The drawing under review shows one solid part. Ordinate dimensions are in mm from its lowest x, y, z. Coordinates: 2 decimals unless noted, no trailing zeros. Order: outer loops, then holes, each group sorted by start corner. A loop starts at its lowest first (then second) coordinate and runs counter-clockwise, first axis right, second up. Notation, with made-up numbers: (-15, 45.5) - (39, 45.5) arc R19 cw to (39, 50.5) - close; hole circle Ø9 at (61.5, 78.5). An arc over 180 degrees is marked (long way). Answer in a Markdown table with one row per item.
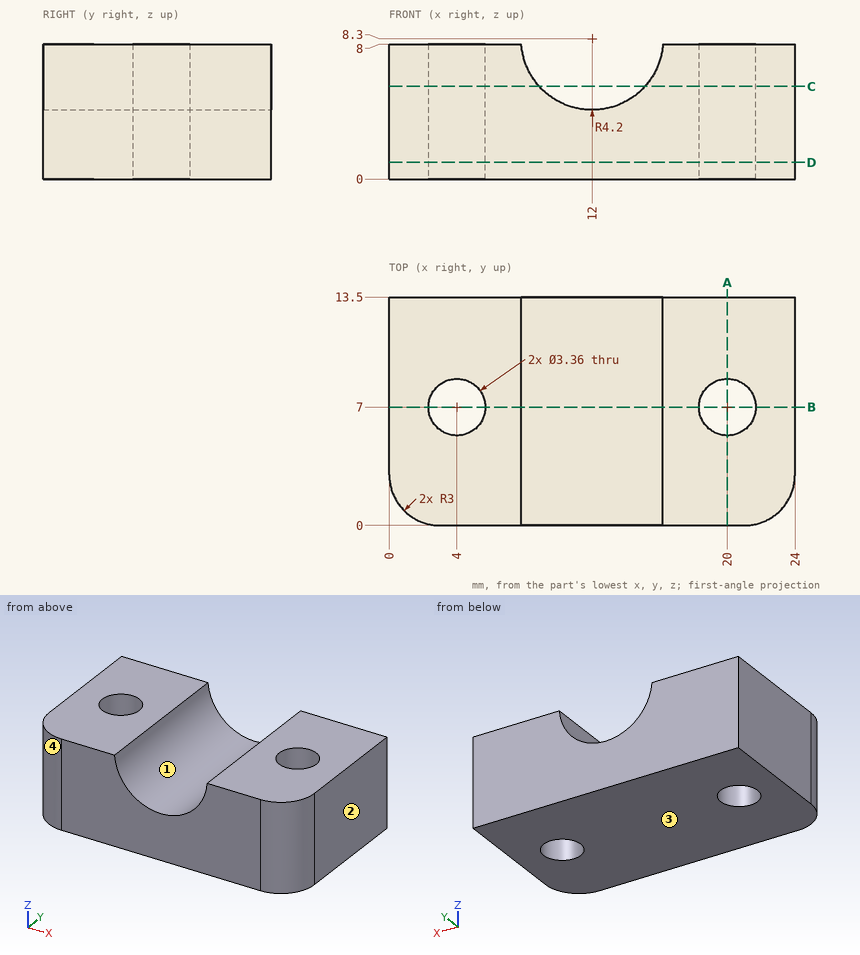
Item 1: Mouldability with a two-part tool opening along X and no side actions: class the marked faces 1, 2, 3 and 4 as +X half, -X half, draft (parallel to the pull), parting line (faces both ways), or undercut.
Check values:
| item | result |
|---|---|
| face 1 | undercut |
| face 2 | +X half |
| face 3 | draft |
| face 4 | -X half |
Item 2: To check wall thickness, follow line 1 (X direction, y = 7, z = 4); line 2 (X direction, y = 6.5, z = 2.5); line 3 (X direction, y = 7.5, z = 6.25). State the ranges of each line that lie inside material, in increasing order. Write a range as from..to.
Check values:
| item | result |
|---|---|
| line 1 | 0..2.32, 5.68..18.32, 21.68..24 |
| line 2 | 0..2.4, 5.6..18.4, 21.6..24 |
| line 3 | 0..2.4, 5.6..8.33, 15.67..18.4, 21.6..24 |
Item 3: We need section B-B, the plane y = 7. Write out the cut boundary in (x, z).
Check values:
| item | result |
|---|---|
| outline | (0, 0) - (2.32, 0) - (2.32, 8) - (0, 8) - close; (5.68, 0) - (18.32, 0) - (18.32, 8) - (16.19, 8) arc R4.2 cw to (7.81, 8) - (5.68, 8) - close; (21.68, 0) - (24, 0) - (24, 8) - (21.68, 8) - close |
Item 4: We need section D-D, the plane z = 1. Write out the cut boundary in (x, y), then the cut area to 3 significant figures.
Check values:
| item | result |
|---|---|
| outline | (0, 3) arc R3 ccw to (3, 0) - (21, 0) arc R3 ccw to (24, 3) - (24, 13.5) - (0, 13.5) - close; hole circle Ø3.36 at (4, 7); hole circle Ø3.36 at (20, 7) |
| area | 302 mm^2 |
Item 5: We need section A-A, the plane x = 20. Write out the cut boundary in (y, z).
Check values:
| item | result |
|---|---|
| outline | (0, 0) - (5.32, 0) - (5.32, 8) - (0, 8) - close; (8.68, 0) - (13.5, 0) - (13.5, 8) - (8.68, 8) - close |
Item 6: We need section C-C, the plane z = 5.5. Write out the cut boundary in (x, y), then the cut area to 3 significant figures.
Check values:
| item | result |
|---|---|
| outline | (0, 3) arc R3 ccw to (3, 0) - (8.87, 0) - (8.87, 13.5) - (0, 13.5) - close; (15.13, 0) - (21, 0) arc R3 ccw to (24, 3) - (24, 13.5) - (15.13, 13.5) - close; hole circle Ø3.36 at (4, 7); hole circle Ø3.36 at (20, 7) |
| area | 218 mm^2 |
